```python
from build123d import *

# Parameters (mm, degrees)
F1_DEPTH  = 107.95
F3_R      = 1.5875
F2_R      = 1.905
F4_DEPTH  = 25.4
F5_SIZE2  = 1.4351924041
F5_SIZE   = 1.651
F7_DEPTH  = 107.95
F8_R      = 1.905
F9_DEPTH  = 25.4
F10_SIZE2 = 1.6559912355
F10_SIZE  = 1.905
F11_R     = 5.08


with BuildPart() as f1:
    # F0 (on Front) → F1 (new body)
    with BuildSketch(Plane.XZ):
        with BuildLine():
            Line((3.175, 0), (0, 0))
            Line((0, 0), (0, -28.575))
            ThreePointArc((0, -28.575), (0.9299359697, -30.8200640303), (3.175, -31.75))
            Line((3.175, -31.75), (22.225, -31.75))
            ThreePointArc((22.225, -31.75), (24.4700640303, -30.8200640303), (25.4, -28.575))
            Line((25.4, -28.575), (25.4, -15.875))
            ThreePointArc((25.4, -15.875), (23.8125, -14.2875), (22.225, -15.875))
            Line((22.225, -15.875), (22.225, -19.05))
            ThreePointArc((22.225, -19.05), (12.7, -28.575), (3.175, -19.05))
            Line((3.175, -19.05), (3.175, 0))
        make_face()
    extrude(amount=F1_DEPTH)

    # F3
    f3_edges = [f1.edges().sort_by_distance(p)[0] for p in [
        (1.5875, 0, 0),
        (1.5875, -107.95, 0),
    ]]
    fillet(f3_edges, radius=F3_R)

    # F2 (on face) → F4 (cut)
    with BuildSketch(Plane(origin=(0, 0, 0), x_dir=(0, -1, 0), z_dir=(-1, 0, 0))):
        with Locations((9.525, -5.08)):
            Circle(F2_R)
        with Locations((98.425, -5.08)):
            Circle(F2_R)
    extrude(amount=-F4_DEPTH, mode=Mode.SUBTRACT)

    # F5
    f5_edges = [f1.edges().sort_by_distance(p)[0] for p in [
        (3.175, -96.52, -5.08),
        (3.175, -7.62, -5.08),
    ]]
    chamfer(f5_edges, length=F5_SIZE, length2=F5_SIZE2)

    # F6 (on face) → F7 (join, through all)
    with BuildSketch(Plane.XZ.offset(107.95)):
        with BuildLine():
            Line((3.175, 0), (0, 0))
            Line((0, 0), (0, -28.575))
            ThreePointArc((0, -28.575), (0.9299359697, -30.8200640303), (3.175, -31.75))
            Line((3.175, -31.75), (22.225, -31.75))
            ThreePointArc((22.225, -31.75), (24.4700640303, -30.8200640303), (25.4, -28.575))
            Line((25.4, -28.575), (25.4, -15.875))
            ThreePointArc((25.4, -15.875), (23.8125, -14.2875), (22.225, -15.875))
            Line((22.225, -15.875), (22.225, -19.05))
            ThreePointArc((22.225, -19.05), (12.7, -28.575), (3.175, -19.05))
            Line((3.175, -19.05), (3.175, 0))
        make_face()
        with BuildLine():
            Line((0, -28.575), (0, 0))
            Line((0, 0), (-1.27, 0))
            Line((-1.27, 0), (-1.27, -28.575))
            ThreePointArc((-1.27, -28.575), (0.0319103576, -31.7180896424), (3.175, -33.02))
            Line((3.175, -33.02), (22.225, -33.02))
            ThreePointArc((22.225, -33.02), (25.3680896424, -31.7180896424), (26.67, -28.575))
            Line((26.67, -28.575), (26.67, -15.875))
            ThreePointArc((26.67, -15.875), (24.4475, -13.6525), (22.225, -15.875))
            ThreePointArc((22.225, -15.875), (23.8125, -14.2875), (25.4, -15.875))
            Line((25.4, -15.875), (25.4, -28.575))
            ThreePointArc((25.4, -28.575), (24.4700640303, -30.8200640303), (22.225, -31.75))
            Line((22.225, -31.75), (3.175, -31.75))
            ThreePointArc((3.175, -31.75), (0.9299359697, -30.8200640303), (0, -28.575))
        make_face()
    extrude(amount=-F7_DEPTH)

    # F8 (on face) → F9 (cut)
    with BuildSketch(Plane(origin=(-1.27, 0, 0), x_dir=(0, -1, 0), z_dir=(-1, 0, 0))):
        with Locations((9.525, -5.08)):
            Circle(F8_R)
        with Locations((98.425, -5.08)):
            Circle(F8_R)
    extrude(amount=-F9_DEPTH, mode=Mode.SUBTRACT)

    # F10
    f10_edges = [f1.edges().sort_by_distance(p)[0] for p in [
        (3.175, -96.52, -5.08),
        (3.175, -7.62, -5.08),
    ]]
    chamfer(f10_edges, length=F10_SIZE, length2=F10_SIZE2)

    # F11
    f11_edges = [f1.edges().sort_by_distance(p)[0] for p in [
        (0.9525, -107.95, 0),
        (0.9525, 0, 0),
    ]]
    fillet(f11_edges, radius=F11_R)


solid = f1.part
```
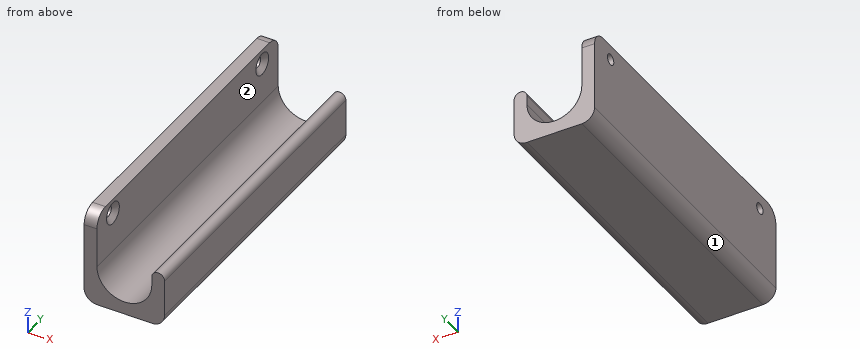
Verification items for the finished model (mm, model axes). Face numbers are marked on the shaded views. A direction names the side the tool comes from. Give positions to 0.01 mm unless a question says otherwise; leave off trailing zeros. Order: outer loops, then holes, each group sorted by start corner. A loop starts at its lowest first (then second) coordinate and runs counter-clockwise, first axis right, second up. Notation, with made-up numbers: M -14.75,22 L -5.75,22 A11 ccw -5.75,26 Z; hole C -17.75,33.25 d11. An arc over 180 degrees is marked long. Return JSON: item names as keys, results as strings. Group by question number.
1) Section check C-C on x = 12.7. Record the cut outline in (y, z) (3 decimals).
2) Go/stop test with flat-tipped pins: pin 1 Ø8 at (x, y) = (13.5, -35.5) entering from +Z; pin 2 Ø5.5 at (y, z) = (-47.5, -10) entering from +X (3 decimals); pin 3 Ø12 at (x, z) = (19.5, -15) entering from +Y; pin 4 Ø1 at (x, y) = (11.5, -57) entering from +Z. Record where each tip stops, or that it passes through.
3) Section check D-D on z = -26.5. Record the cut outline in (x, y), and give its area (3 significant figures).
4) Scan lines: line 1 (X direction, y = -43, z = -13) (3 decimals); line 2 (Z direction, x = 12.25, y = -55); line 3 (X direction, y = -25, z = -22.5). Record each from-to range of solid material in increasing order.
5) Section check A-A on z = -17. Record the cut outline in (x, y) (3 decimals), and give its area (3 significant figures).
6) Access from +Z, -Z, +X, -X, +Y, -Y to the whole of each face (thin tool, end or side, straight path). Record for the marked faces 1 and 2.
Answer block:
{
 "1": {"outline": "M -107.95,-33.02 L 0,-33.02 L 0,-28.575 L -107.95,-28.575 Z"},
 "2": {"pin 1": "stops at z = -27.28", "pin 2": "stops at x = 3.175", "pin 3": "stops at y = 0", "pin 4": "stops at z = -28.42"},
 "3": {"outline": "M -1.27,-107.95 L 6.77,-107.95 L 6.77,0 L -1.27,0 Z; M 18.63,-107.95 L 26.67,-107.95 L 26.67,0 L 18.63,0 Z", "area": "1,730 mm^2"},
 "4": {"line 1": "x = -1.27 to 3.175", "line 2": "z = -33.02 to -28.56", "line 3": "x = -1.27 to 3.82, 21.58 to 26.67"},
 "5": {"outline": "M -1.27,-107.95 L 3.175,-107.95 L 3.175,0 L -1.27,0 Z; M 22.225,-107.95 L 26.67,-107.95 L 26.67,0 L 22.225,0 Z", "area": "960 mm^2"},
 "6": {"face 1": "-Z, -X, +Y, -Y", "face 2": "+Z, +Y, -Y"}
}
